Check sheet for the modelled part. Datum: model origin and axes. Units: mm. Face numbers are marked on the shaded views. A direction names the side the tool comes from. Round coordinates to 2 decimals unless told otherwise and drop trailing zeros. Write each loop counter-clockwise with the first axis right and the second up, starting at its lowest first coordinate (ties: lowest second). Pieces come first, ordered by that corner, then holes. Notation, with made-up numbers: M 9,-6 L 54,-6 A21 cw 54,-2 Z; hole C 52.5,45 d4. An arc over 180 degrees is marked long. Answer in a Markdown table with one row per item.
```python
from build123d import *

# Parameters (mm, degrees)
SKETCH_1_W        = 9.5
SKETCH_1_H        = 20
SKETCH_2_R        = 1
EXTRUDE_457_DEPTH = 15
SKETCH_3_W        = 2
SKETCH_3_H        = 10
EXTRUDE_556_DEPTH = 5


with BuildPart() as part:
    # Эскиз1 → Revolve 326 (revolve)
    with BuildSketch(Plane.XY, mode=Mode.PRIVATE) as revolve_326_sk:
        with Locations((4.75, 10)):
            Rectangle(SKETCH_1_W, SKETCH_1_H)
    revolve(revolve_326_sk.sketch.rotate(Axis((0, 0, 0), (0, 1, 0)), 90), axis=Axis((0, 0, 0), (0, 1, 0)))

    # Эскиз2 → Extrude 457 (add)
    with BuildSketch(Plane(origin=(0, 0, 0), x_dir=(1, 0, 0), z_dir=(0, 1, 0))):
        with Locations(Location((0, -3, 0), (0, 0, 270))):
            Circle(SKETCH_2_R)
        with Locations(Location((0, 3, 0), (0, 0, 270))):
            Circle(SKETCH_2_R)
    extrude(amount=-EXTRUDE_457_DEPTH)

    # Эскиз3 → Extrude 556 (add)
    with BuildSketch(Plane(origin=(0, 0, 0), x_dir=(1, 0, 0), z_dir=(0, 1, 0))):
        Rectangle(SKETCH_3_W, SKETCH_3_H)
    extrude(amount=-EXTRUDE_556_DEPTH)


solid = part.part
```
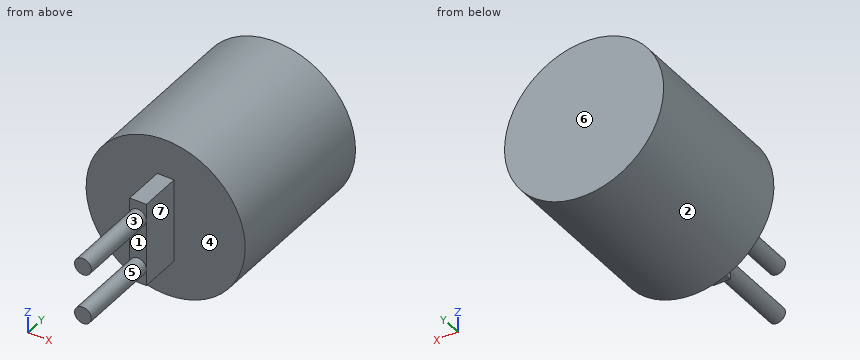
1. Access from +Z, -Z, +X, -X, +Y, -Y to the whole of each face (thin tool, end or side, straight path). Record for the marked faces 5, 6 and 7.
Found:
| item | result |
|---|---|
| face 5 | -Y |
| face 6 | +Z, -Z, +X, -X, +Y |
| face 7 | +Z, -Z, +X, -Y |
2. Section check B-B, the plane z = 0. Record the cut outline in (x, y), and give its area (3 significant figures).
Found:
| item | result |
|---|---|
| outline | M -9.5,0 L -1,0 L -1,-5 L 1,-5 L 1,0 L 9.5,0 L 9.5,20 L -9.5,20 Z |
| area | 390 mm2 |
3. Scan lines: L1, parallel to Y at x = 7.5, z = 2; L2, parallel to Z at x = 0, y = -12; L3, parallel to Z at x = 1, y = 4.5. Record each from-to range of solid material in increasing order.
Found:
| item | result |
|---|---|
| L1 | y = 0 to 20 |
| L2 | z = -4 to -2, 2 to 4 |
| L3 | z = -9.45 to 9.45 |
4. Draft check along Z on the marked faces 1, 2, 3 and 4. Enter one of: +Z half, -Z half, draft (parallel to the pull), parting line (faces both ways), or undercut.
Found:
| item | result |
|---|---|
| face 1 | undercut |
| face 2 | parting line |
| face 3 | undercut |
| face 4 | draft |
5. Section check D-D, the plane z = -3.5. Record the cut outline in (x, y).
Found:
| item | result |
|---|---|
| outline | M -8.83,0 L -1,0 L -1,-5 L -0.87,-5 L -0.87,-15 L 0.87,-15 L 0.87,-5 L 1,-5 L 1,0 L 8.83,0 L 8.83,20 L -8.83,20 Z |
6. Section check C-C, the plane y = 9. Record the cut outline in (x, z), and give its area (3 significant figures).
Found:
| item | result |
|---|---|
| outline | C 0,0 d19 |
| area | 284 mm2 |
7. Go/stop test with flat-tipped pins: pin 1 (5 mm diameter, centred on x = 6, y = 11.5, fed in from -Z); pin 2 (2.5 mm diameter, centred on y = -2, z = -1.5, fed in from +X); pin 3 (1.5 mm diameter, centred on x = 6, y = 8.5, fed in from +Z); pin 4 (1.5 mm diameter, centred on y = -10.5, z = -5, fed in from -X). Record where each tip stops, or that it passes through.
Found:
| item | result |
|---|---|
| pin 1 | stops at z = -8.83 |
| pin 2 | stops at x = 1 |
| pin 3 | stops at z = 7.92 |
| pin 4 | passes through |
8. Section check A-A, the plane x = 0. Record the cut outline in (y, z), and give its area (3 significant figures).
Found:
| item | result |
|---|---|
| outline | M -15,-4 L -5,-4 L -5,-5 L 0,-5 L 0,-9.5 L 20,-9.5 L 20,9.5 L 0,9.5 L 0,5 L -5,5 L -5,4 L -15,4 L -15,2 L -5,2 L -5,-2 L -15,-2 Z |
| area | 470 mm2 |
